Could you check a few things on this model? Use its own coordinates, in mm. Give positions to 0.01 mm unless a question says otherwise; leave off trailing zeros. Order: outer loops, then holes, each group sorted by start corner. A loop starts at its lowest first (then second) coordinate and runs counter-clockwise, first axis right, second up. Notation, with made-up numbers: M 30,-36 L 61,-36 A21 ccw 61,-21 Z; hole C -12.75,36.25 d3. An arc over 180 degrees is marked long. Use a Markdown table: item, result. Add a question column.
Item 1: Suppose I cut it at B-B on x = -37. Write out the boundary of the cut face in (y, z), plus the area to 3 significant figures.
Item 2: Suppose I cut it at A-A on y = -51.25. Write out the boundary of the cut face in (x, z).
Item 3: Suppose I cut it at C-C on z = 1.75. Write out the boundary of the cut face in (x, y).
Item 4: If I drill on L1, parallel to Y at x = 1.5, z = 0.25; L2, parallel to X at y = -52.25, z = 0.8; L3, parallel to Y at x = -49, z = 0.4, over which ranges is the centre line in solid material (lowest first)? Write a range as from..to.
from build123d import *

# Parameters (mm, degrees)
ESQUISSE9_R        = 1.5
ESQUISSE9_R_2      = 3.75
ESQUISSE9_W        = 9
ESQUISSE9_H        = 3
ESQUISSE9_W_2      = 8
BOSS_EXTRU_9_DEPTH = 3


with BuildPart() as part:
    # Esquisse9 → Boss.-Extru.9 (new body)
    with BuildSketch(Plane.XY):
        with BuildLine():
            Line((-63.040292512, -47.505063948), (16.959707488, -47.505063948))
            ThreePointArc((16.959707488, -47.505063948), (22.959707488, -53.505063948), (16.959707488, -59.505063948))
            Line((16.959707488, -59.505063948), (-63.040292512, -59.505063948))
            ThreePointArc((-63.040292512, -59.505063948), (-69.040292512, -53.505063948), (-63.040292512, -47.505063948))
        make_face()
        with Locations((-15.040292512, -53.505063948)):
            Circle(ESQUISSE9_R, mode=Mode.SUBTRACT)
        with Locations((16.959707488, -53.505063948)):
            Circle(ESQUISSE9_R, mode=Mode.SUBTRACT)
        with Locations((-63.040292512, -53.505063948)):
            Circle(ESQUISSE9_R_2, mode=Mode.SUBTRACT)
        with Locations((-35.540292512, -53.505063948)):
            Rectangle(ESQUISSE9_W, ESQUISSE9_H, mode=Mode.SUBTRACT)
        with Locations((2.959707488, -53.505063948)):
            Rectangle(ESQUISSE9_W_2, ESQUISSE9_H, mode=Mode.SUBTRACT)
        with BuildLine():
            Line((-53.040292512, -52.505063948), (-48.040292512, -52.505063948))
            ThreePointArc((-48.040292512, -52.505063948), (-47.040292512, -53.505063948), (-48.040292512, -54.505063948))
            Line((-48.040292512, -54.505063948), (-53.040292512, -54.505063948))
            ThreePointArc((-53.040292512, -54.505063948), (-54.040292512, -53.505063948), (-53.040292512, -52.505063948))
        make_face(mode=Mode.SUBTRACT)
    extrude(amount=BOSS_EXTRU_9_DEPTH)


solid = part.part
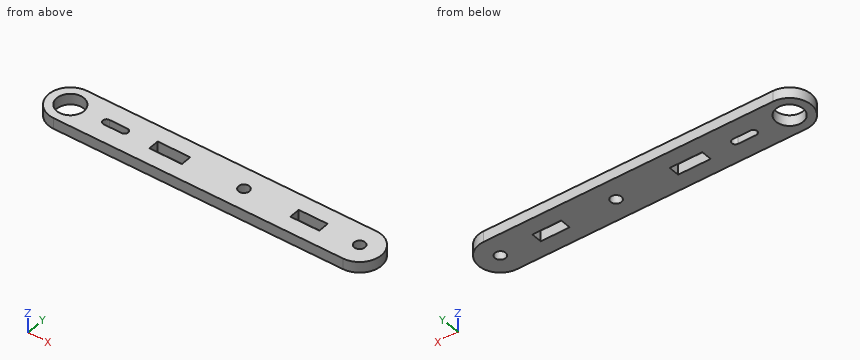
Findings below:
| question | item | result |
|---|---|---|
| 1 | outline | M -59.51,0 L -55.01,0 L -55.01,3 L -59.51,3 Z; M -52.01,0 L -47.51,0 L -47.51,3 L -52.01,3 Z |
| 1 | area | 27.0 mm^2 |
| 2 | outline | M -68.6,0 L -66.04,0 L -66.04,3 L -68.6,3 Z; M -60.04,0 L 22.52,0 L 22.52,3 L -60.04,3 Z |
| 3 | outline | M -63.04,-59.51 L 16.96,-59.51 A6 ccw 16.96,-47.51 L -63.04,-47.51 A6 ccw Z; hole C -63.04,-53.51 d7.5; hole M -53.04,-54.51 L -48.04,-54.51 A1 ccw -48.04,-52.51 L -53.04,-52.51 A1 ccw Z; hole M -40.04,-55.01 L -31.04,-55.01 L -31.04,-52.01 L -40.04,-52.01 Z; hole C -15.04,-53.51 d3; hole M -1.04,-55.01 L 6.96,-55.01 L 6.96,-52.01 L -1.04,-52.01 Z; hole C 16.96,-53.51 d3 |
| 4 | L1 | y = -59.51..-55.01, -52.01..-47.51 |
| 4 | L2 | x = -68.91..-66.57, -59.51..-40.04, -31.04..-15.86, -14.22..-1.04, 6.96..16.14, 17.78..22.83 |
| 4 | L3 | y = -59.51..-54.51, -52.51..-47.51 |
